Source: CAD feature listing. Evaluate the final solid. Frame: model axes, mm. A direction names the side the tool comes from. Give positions to 0.01 mm unless a question says otherwise; leave off trailing zeros. Order: outer loops, then holes, each group sorted by start corner. A loop starts at its lowest first (then second) coordinate and runs counter-clockwise, first axis right, second up. Notation, with made-up numbers: M -32,52.25 L 15,52.25 A19 cw 15,60.25 Z; hole C 19.25,22 d9. An arc over 180 degrees is marked long. Use CSV: the item, a comma, the result in double quotes. Start each with the question number.
1. Section query A-A, the plane y = 0. State how many separate pieces and enclosed holes the cut face has, plus the area to 3 significant figures.
2. Section query D-D, the plane x = 11. Return the cut outline in (y, z), plus the area to 3 significant figures.
3. Mould query, pull axis Y, two halves, no side actions, for faces 4 (the cylindrical face through (37.935, 5.416, -3.787)), 5 (the flat face through (4, -11.43, 5)), 6 (the flat face through (43, 0, 3)). Classes: released by +Y, released by -Y, zero draft, split by the parting line, or undercut.
4. Section query C-C, the plane x = 42. Return the cut outline in (y, z), plus the area to 3 significant figures.
5. Pin query (flat end, axial travel): P1, Ø3, axis at x = 31.5, y = -9.5, coming from the -Z side; P2, Ø3, axis at y = 8, z = -6.5, coming from the +X side; P3, Ø1.4, axis at y = -1.5, z = 13.5, coming from the +X side (3 decimals). Return the tip coordinate at first contact, or that it passes through.
6. Line query: line 1 along Y through (x, z) = (10, -8); line 2 along Z through (x, y) = (5.5, 7.5); line 3 along X through (y, z) = (-15.5, 0.5). Output: solid intervals per line, ascending. Write a range as [from, to].
7. Reachability of faces 1 (the cylindrical face through (3.131, -6.267, -5.287)), 2 (the flat face through (4, -11.43, -5)), 3 (the flat face through (33.15, -4, 7)) from +Z, -Z, +X, -X, +Y, -Y: full face, straight path, thin tool, end or side. Return the list, or none.
8. Section query B-B, the plane x = 3.8. Return the cut outline in (y, z), plus the area to 3 significant figures.
from build123d import *

# Parameters (mm, degrees)
SKETCH2_R          = 1.25
CUT_EXTRUDE1_DEPTH = 6.35
SKETCH3_R          = 1.5
CUT_EXTRUDE2_DEPTH = 6.35
CUT_EXTRUDE5_START = 17.78
CUT_EXTRUDE5_DEPTH = 6.35
SKETCH4_R          = 4
CUT_EXTRUDE3_DEPTH = 6.8
CIRPATTERN1_COUNT  = 4
CUT_EXTRUDE4_DEPTH = 3.175
CIRPATTERN2_COUNT  = 6


with BuildPart() as part:
    # Sketch1 → Revolve1 (revolve)
    with BuildSketch(Plane.XY):
        Polygon((0, 0), (0, 15.865968489), (7.5, 17.5), (34.951150155, 17.5), (39.5, 15.865968489), (39.5, 6.346727069), (43, 6.346727069), (43, 2.5), (59.5, 2.5), (59.5, 0), align=None)
    revolve(axis=Axis((59.5, 0, 0), (-1, 0, 0)))

    # Sketch2 → Cut-Extrude1 (cut)
    with BuildSketch(Plane(origin=(39.5, 0, 0), x_dir=(0, 0, -1), z_dir=(1, 0, 0))):
        with Locations((0, 8.5)):
            Circle(SKETCH2_R)
        with Locations((7.361215932, -4.25)):
            Circle(SKETCH2_R)
        with Locations((-7.361215932, -4.25)):
            Circle(SKETCH2_R)
    extrude(amount=-CUT_EXTRUDE1_DEPTH, mode=Mode.SUBTRACT)

    # Sketch3 → Cut-Extrude2 (cut)
    with BuildSketch(Plane.ZY):
        with Locations((-8.838834765, 8.838834765)):
            Circle(SKETCH3_R)
        with Locations((8.838834765, -8.838834765)):
            Circle(SKETCH3_R)
        with Locations((6.717514421, 6.717514421)):
            Circle(SKETCH3_R)
        with Locations((-6.717514421, -6.717514421)):
            Circle(SKETCH3_R)
    extrude(amount=-CUT_EXTRUDE2_DEPTH, mode=Mode.SUBTRACT)

    # Sketch6 → Cut-Extrude5 (cut)
    with BuildSketch(Plane(origin=(0, 0, 0), x_dir=(1, 0, 0), z_dir=(0, 1, 0)).offset(CUT_EXTRUDE5_START)):
        with BuildLine():
            Line((6.8, 4), (6.8, -4))
            ThreePointArc((6.8, -4), (3.8, -7), (0.8, -4))
            Line((0.8, -4), (0.8, 4))
            ThreePointArc((0.8, 4), (3.8, 7), (6.8, 4))
        make_face()
    cut_extrude5 = extrude(amount=-CUT_EXTRUDE5_DEPTH, mode=Mode.SUBTRACT)

    # Sketch4 → Cut-Extrude3 (cut)
    with BuildSketch(Plane.ZY):
        with Locations((0, 11)):
            Circle(SKETCH4_R)
    cut_extrude3 = extrude(amount=-CUT_EXTRUDE3_DEPTH, mode=Mode.SUBTRACT)

    # CirPattern1: Cut-Extrude5, Cut-Extrude3 ×4 about axis
    cirpattern1_axis = Axis((0, 0, 0), (1, 0, 0))
    for i in range(1, CIRPATTERN1_COUNT):
        add(cut_extrude5.rotate(cirpattern1_axis, i * 360 / CIRPATTERN1_COUNT), mode=Mode.SUBTRACT)
        add(cut_extrude3.rotate(cirpattern1_axis, i * 360 / CIRPATTERN1_COUNT), mode=Mode.SUBTRACT)

    # Sketch5 → Cut-Extrude4 (cut)
    with BuildSketch(Plane(origin=(39.5, 0, 0), x_dir=(0, 0, -1), z_dir=(1, 0, 0))):
        with BuildLine():
            ThreePointArc((2.25, 7.361215932), (3.823598567, 5.40719909), (6.068181818, 6.528020351))
            ThreePointArc((6.068181818, 6.528020351), (18.421673948, 10.753421518), (21.995966692, -1.803935458))
            ThreePointArc((21.995966692, -1.803935458), (19.302148043, 18.245874868), (2.25, 7.361215932))
        make_face()
    cut_extrude4 = extrude(amount=-CUT_EXTRUDE4_DEPTH, mode=Mode.SUBTRACT)

    # CirPattern2: Cut-Extrude4 ×6 about axis
    cirpattern2_axis = Axis((0, 0, 0), (1, 0, 0))
    for i in range(1, CIRPATTERN2_COUNT):
        add(cut_extrude4.rotate(cirpattern2_axis, i * 360 / CIRPATTERN2_COUNT), mode=Mode.SUBTRACT)


solid = part.part
Result set:
1,separate pieces,"3"
1,enclosed holes,"0"
1,area,"1,300 mm2"
2,outline,"C 0,0 d35"
2,area,"962 mm2"
3,face 4,"undercut"
3,face 5,"released by -Y"
3,face 6,"zero draft"
4,outline,"C 0,0 d12.69"
4,area,"127 mm2"
5,P1,"z = -15.56"
5,P2,"x = 39.5"
5,P3,"x = 36.325"
6,line 1,"[-15.56, 15.56]"
6,line 2,"[-15.33, -9.52], [-8.16, -1.94], [1.94, 5.44], [8, 15.33]"
6,line 3,"[0, 0.8], [6.8, 39.5]"
7,face 1,"-X"
7,face 2,"-Y"
7,face 3,"+X"
8,outline,"M -15.16,-7 A16.69 ccw -7,-15.16 L -7,-11.43 L -3.98,-11.43 A4 cw long 3.98,-11.43 L 7,-11.43 L 7,-15.16 A16.69 ccw 15.16,-7 L 11.43,-7 L 11.43,-3.98 A4 cw long 11.43,3.98 L 11.43,7 L 15.16,7 A16.69 ccw 7,15.16 L 7,11.43 L 3.98,11.43 A4 cw long -3.98,11.43 L -7,11.43 L -7,15.16 A16.69 ccw -15.16,7 L -11.43,7 L -11.43,3.98 A4 cw long -11.43,-3.98 L -11.43,-7 Z; hole C -8.84,8.84 d3; hole C -6.72,-6.72 d3; hole C 6.72,6.72 d3; hole C 8.84,-8.84 d3"
8,area,"466 mm2"
